Check sheet for the modelled part. Datum: model origin and axes. Units: mm. A direction names the side the tool comes from. Round coordinates to 2 decimals unless told otherwise and drop trailing zeros. Order: outer loops, then holes, each group sorted by start corner. A loop starts at its lowest first (then second) coordinate and runs counter-clockwise, first axis right, second up. Notation, with made-up numbers: (84, -2.75) -> (120, -2.75) arc R32 cw to (120, 29.25) -> close; hole circle Ø6 at (52.5, 53.5). An arc over 180 degrees is marked (long way). Answer in a Markdown table with one row per item.
```python
from build123d import *

# Parameters (mm, degrees)
SKETCH3_R                = 1
BOSS_EXTRUDE1_DEPTH      = 10
BOSS_EXTRUDE2_DEPTH      = 11.25
BOSS_EXTRUDE2_DEPTH_BACK = 11.25
SKETCH6_R                = 1
BOSS_EXTRUDE3_DEPTH      = 2.8125
BOSS_EXTRUDE3_DEPTH_BACK = 2.8125
SKETCH7_R                = 1
BOSS_EXTRUDE4_DEPTH      = 2.8125


with BuildPart() as part:
    # Sketch3 → Boss-Extrude1 (new body)
    with BuildSketch(Plane(origin=(0, 0, 0), x_dir=(0, 0, -1), z_dir=(1, 0, 0))):
        Circle(SKETCH3_R)
    extrude(amount=-BOSS_EXTRUDE1_DEPTH)

    # Sketch4 → Boss-Extrude2 (add, two sides)
    with BuildSketch(Plane(origin=(0, 0, 0), x_dir=(1, 0, 0), z_dir=(0, 1, 0))) as boss_extrude2_sk:
        with BuildLine():
            ThreePointArc((-9.5, 0), (-9.646446609, 0.353553391), (-10, 0.5))
            Line((-10, 0.5), (-10, -0.5))
            ThreePointArc((-10, -0.5), (-9.646446609, -0.353553391), (-9.5, 0))
        make_face()
        with BuildLine():
            Line((-10, -0.5), (-10, 0.5))
            ThreePointArc((-10, 0.5), (-10.5, 0), (-10, -0.5))
        make_face()
    extrude(amount=BOSS_EXTRUDE2_DEPTH)
    extrude(boss_extrude2_sk.sketch, amount=-BOSS_EXTRUDE2_DEPTH_BACK)

    # Sketch6 → Boss-Extrude3 (add, two sides)
    with BuildSketch(Plane(origin=(0, 0, 0), x_dir=(1, 0, 0), z_dir=(0, 1, 0))) as boss_extrude3_sk:
        with Locations((-10, 0)):
            Circle(SKETCH6_R)
    extrude(amount=BOSS_EXTRUDE3_DEPTH)
    extrude(boss_extrude3_sk.sketch, amount=-BOSS_EXTRUDE3_DEPTH_BACK)

    # Sketch7 → Boss-Extrude4 (add)
    with BuildSketch(Plane(origin=(0, 11.25, 0), x_dir=(1, 0, 0), z_dir=(0, 1, 0))):
        with Locations((-10, 0)):
            Circle(SKETCH7_R)
    boss_extrude4 = extrude(amount=-BOSS_EXTRUDE4_DEPTH)

    # Mirror1: Boss-Extrude4 across plane
    add(boss_extrude4.mirror(Plane.ZX))


solid = part.part
```
(1) Section check A-A on z = 0.75. Record the boundary of the cut face in (x, y), plus the area to 3 significant figures.
Solutions:
| item | result |
|---|---|
| outline | (-10.66, -11.25) -> (-9.34, -11.25) -> (-9.34, -8.44) -> (-10.66, -8.44) -> close; (-10.66, -2.81) -> (-9.34, -2.81) -> (-9.34, -0.66) -> (0, -0.66) -> (0, 0.66) -> (-9.34, 0.66) -> (-9.34, 2.81) -> (-10.66, 2.81) -> close; (-10.66, 8.44) -> (-9.34, 8.44) -> (-9.34, 11.25) -> (-10.66, 11.25) -> close |
| area | 27.2 mm^2 |
(2) Section check D-D on y = -7.25. Record the boundary of the cut face in (x, z), plus the area to 3 significant figures.
Solutions:
| item | result |
|---|---|
| outline | circle Ø1 at (-10, 0) |
| area | 0.785 mm^2 |
(3) Section check B-B on y = 9.5. Record the boundary of the cut face in (x, z), plus the area to 3 significant figures.
Solutions:
| item | result |
|---|---|
| outline | circle Ø2 at (-10, 0) |
| area | 3.14 mm^2 |
(4) Scan lines: probe 1 along Y at (x, z) = (-9.25, -0.3); probe 2 along X at (y, z) = (4, 0.05); probe 3 along Y at (x, z) = (-3, -0.05). Record each from-to range of solid material in increasing order. Write a range as from..to.
Solutions:
| item | result |
|---|---|
| probe 1 | -11.25..-8.44, -2.81..2.81, 8.44..11.25 |
| probe 2 | -10.5..-9.5 |
| probe 3 | -1..1 |
(5) Depth check by flat-ended pin: pin 1 Ø5 at (x, y) = (-7.5, -3.5) entering from -Z. Enter the tip coordinate at first touch or a pass-through.
Solutions:
| item | result |
|---|---|
| pin 1 | z = -1 |
(6) Draft check along Y on faces 4 (the flat face through (-10, -11.25, 0)), 5 (the flat face through (-10, 11.25, 0)), 6 (the flat face through (0, 0, 0)), 7 (the cylindrical face through (-5, -1, 0)). Enter one of: pulls with the +Y half, pulls with the -Y half, needs draft (parallel to the pull), parting line crosses it, or undercut.
Solutions:
| item | result |
|---|---|
| face 4 | pulls with the -Y half |
| face 5 | pulls with the +Y half |
| face 6 | needs draft |
| face 7 | parting line crosses it |
(7) Tool access check on faces 1 (the cylindrical face through (-10.8, 9.9, 0.6)), 2 (the cylindrical face through (-10.8, -9.9, 0.6)), 3 (the cylindrical face through (-11, 0, 0)). Record the directions out of +Z, -Z, +X, -X, +Y, -Y that give a thin tool (end or side, any length) a straight path to the whole face; none if there is none.
Solutions:
| item | result |
|---|---|
| face 1 | +Y |
| face 2 | -Y |
| face 3 | none |
(8) Section check C-C on x = -5.5. Record the boundary of the cut face in (y, z), plus the area to 3 significant figures.
Solutions:
| item | result |
|---|---|
| outline | circle Ø2 at (0, 0) |
| area | 3.14 mm^2 |
